Model file for the job. Use its own axes, mm. A direction names the side the tool comes from. Coordinates: 2 decimals unless noted, no trailing zeros. Write each loop counter-clockwise with the first axis right and the second up, starting at its lowest first coordinate (ties: lowest second). Pieces come first, ordered by that corner, then holes. Notation, with made-up numbers: M 9,19 L 27,19 A16 cw 27,28 Z; hole C -15.75,-24 d10. An arc over 180 degrees is marked long. Use CSV: the item, a comma, the result in double quotes. Start each with the question number.
Autodesk Inventor part; units mm, degrees
ref_plane "YZ Plane" through (0, 0, 0) normal (1, 0, 0) x (0, 1, 0)
ref_plane "XZ Plane" through (0, 0, 0) normal (0, 1, 0) x (-1, 0, 0)
ref_plane "XY Plane" through (0, 0, 0) normal (0, 0, 1) x (1, 0, 0)
sketch "Esquisse1" plane through (0, 0, 0) normal (1, 0, 0) x (0, 1, 0)
  line L0 (0, 0) -> (58, 0)
  line L1 (58, 0) -> (58, -58)
  line L2 (58, -58) -> (0, -58)
  line L3 (0, -58) -> (0, 0)
  line L4 (50, 0) -> (58, 0)
  line L5 (58, 0) -> (58, -6)
  line L6 (58, -6) -> (50, -6)
  line L7 (50, -6) -> (50, 0)
  line L8 (58, -52) -> (50, -52)
  line L9 (50, -52) -> (50, -58)
  line L10 (50, -58) -> (58, -58)
  line L11 (58, -58) -> (58, -52)
  dimension "d0" = 58
  dimension "d1" = 58
  dimension "d2" = 6
  dimension "d3" = 8
  dimension "d4" = 8
  dimension "d5" = 6
  dimension "d15" = 46
extrude "Extrusion1" add sketch "Esquisse1" along normal blind 6 contours L0 L7 L6 L1 L8 L9 L2 L3
sketch "Esquisse2" plane through (0, 50, -6) normal (0, 0, 1) x (1, 0, 0)
  circle A0 centre (3, 5) radius 1.5
  line L0 (6, 8) -> (6, 0)
  line L1 (0, 8) -> (0, 0)
  line L2 (0, 0) -> (6, 0)
  line L3 (0, 8) -> (6, 8)
  point P0 (0, -50)
  dimension "d8" = 3
  dimension "d9" = 6
  dimension "d10" = 8
  dimension "d11" = 3
  dimension "d32" = 3
extrude "Extrusion2" cut sketch "Esquisse2" against normal up to next contours A0
sketch "Esquisse3" plane through (6, 0, 0) normal (1, 0, 0) x (0, 0, -1)
  line L0 (16.5, 15) -> (21.5, 15)
  line L1 (21.5, 15) -> (21.5, 35)
  line L2 (21.5, 35) -> (16.5, 35)
  line L3 (16.5, 35) -> (16.5, 15)
  line L4 (0, 50) -> (0, 0)
  line L5 (0, 0) -> (58, 0)
  line L6 (6, 50) -> (0, 50)
  dimension "d16" = 5
  dimension "d17" = 20
  dimension "d18" = 16.5
  dimension "d19" = 15
  dimension "d20" = 50
  dimension "d21" = 58
extrude "Extrusion3" add sketch "Esquisse3" along normal blind 15
sketch "Esquisse4" plane through (6, 15, -16.5) normal (0, 0, 1) x (1, 0, 0)
  circle A0 centre (7.5, 10) radius 2.5
  line L0 (0, 20) -> (15, 20)
  line L1 (0, 0) -> (15, 0)
  line L2 (15, 20) -> (15, 0)
  line L3 (0, 35) -> (0, -15)
  point P0 (-6, -15)
  dimension "d24" = 5
  dimension "d25" = 20
  dimension "d26" = 15
  dimension "d27" = 7.5
  dimension "d28" = 10
extrude "Extrusion4" cut sketch "Esquisse4" against normal up to next contours A0
fillet "Congé1" radius 3 2 edges at (6, 58, -29) (0, 58, -29)
equation "\"d5\" = d2"
equation "\"d11\" = 0.5 * d9"
equation "\"d19\" = 0.5 * d20 - 0.5 * d17"
equation "\"d27\" = 0.5 * d26"
equation "\"d28\" = 0.5 * d25"
properties part number "membre_pince" material "Plastique PC/ABS"
1) Band-saw the part on D-D on x = 8. List the corners of the cut face in (y, z), then the cut area to 3 significant figures.
2) Band-saw the part on B-B on x = 13.5. List the corners of the cut face in (y, z).
3) Tool access for faces 1 (the face through (3, 53, -6)), 2 (the face through (3, 53, -52)), 3 (the face through (11.7, 22.6, -21.5)), 4 (the face through (13, 15, -19)), 5 (the face through (11.7, 27.4, -16.5)): list every direction of +Z, -Z, +X, -X, +Y, -Y with a clear straight run to the whole face (end or side of a thin tool).
4) Drop flat-ended pins along their axis: P1, Ø6.5, axis at x = 13.5, y = 25, coming from the +Z side; P2, Ø3, axis at x = 4, y = 53.5, coming from the -Z side; P3, Ø2.5, axis at x = 13, z = -18.5, coming from the +Y side. Give the stop position or say it passes through.
5) Band-saw the part on C-C on y = 19. List the corners of the cut face in (x, z), then the cut area to 3 significant figures.
6) Wall check: L1, parallel to Y at x = 3, z = -40; L2, parallel to Y at x = 13.5, z = -19.2; L3, parallel to X at y = 25, z = -33.5. Give the ranges that are in metal, low to high. Write a range as [from, to].
Findings below:
1,outline,"M 15,-21.5 L 35,-21.5 L 35,-16.5 L 15,-16.5 Z"
1,area,"100 mm2"
2,outline,"M 15,-21.5 L 22.5,-21.5 L 22.5,-16.5 L 15,-16.5 Z; M 27.5,-21.5 L 35,-21.5 L 35,-16.5 L 27.5,-16.5 Z"
3,face 1,"+Z, +X, -X, +Y"
3,face 2,"-Z, +X, -X, +Y"
3,face 3,"-Z, +X, +Y, -Y"
3,face 4,"+Z, -Z, +X, -Y"
3,face 5,"+Z, +X, +Y, -Y"
4,P1,"stops at z = -16.5"
4,P2,"stops at z = -52"
4,P3,"stops at y = 35"
5,outline,"M 0,-58 L 6,-58 L 6,-21.5 L 21,-21.5 L 21,-16.5 L 6,-16.5 L 6,0 L 0,0 Z"
5,area,"423 mm2"
6,L1,"y = [0, 53.5], [56.5, 58]"
6,L2,"y = [15, 22.5], [27.5, 35]"
6,L3,"x = [0, 6]"
